from build123d import *

# Parameters (mm, degrees)
F0_W     = 457.2
F0_H     = 304.8
F0_R     = 1.8288
F0_R_2   = 41.34485
F1_DEPTH = 12.7
F2_W     = 144.399
F2_H     = 82.042
F3_DEPTH = 3.175
F4_R     = 1.5875
F5_DEPTH = 3.175


with BuildPart() as f1:
    # F0 (on Top) → F1 (new body)
    with BuildSketch(Plane.XY):
        Rectangle(F0_W, F0_H)
        with Locations((-186.120166, -107.938549)):
            Circle(F0_R, mode=Mode.SUBTRACT)
        with Locations((-98.490166, -107.938549)):
            Circle(F0_R, mode=Mode.SUBTRACT)
        with Locations((-142.305166, -64.123549)):
            Circle(F0_R_2, mode=Mode.SUBTRACT)
        with Locations((-186.120166, -20.308549)):
            Circle(F0_R, mode=Mode.SUBTRACT)
        with Locations((-98.490166, -20.308549)):
            Circle(F0_R, mode=Mode.SUBTRACT)
        with Locations((98.490166, -107.938549)):
            Circle(F0_R, mode=Mode.SUBTRACT)
        with Locations((186.120166, -107.938549)):
            Circle(F0_R, mode=Mode.SUBTRACT)
        with Locations((98.490166, -20.308549)):
            Circle(F0_R, mode=Mode.SUBTRACT)
        with Locations((142.305166, -64.123549)):
            Circle(F0_R_2, mode=Mode.SUBTRACT)
        with Locations((186.120166, -20.308549)):
            Circle(F0_R, mode=Mode.SUBTRACT)
        with Locations((-186.120166, 20.308549)):
            Circle(F0_R, mode=Mode.SUBTRACT)
        with Locations((-142.305166, 64.123549)):
            Circle(F0_R_2, mode=Mode.SUBTRACT)
        with Locations((-98.490166, 20.308549)):
            Circle(F0_R, mode=Mode.SUBTRACT)
        with Locations((-186.120166, 107.938549)):
            Circle(F0_R, mode=Mode.SUBTRACT)
        with Locations((-98.490166, 107.938549)):
            Circle(F0_R, mode=Mode.SUBTRACT)
        with Locations((98.490166, 20.308549)):
            Circle(F0_R, mode=Mode.SUBTRACT)
        with Locations((186.120166, 20.308549)):
            Circle(F0_R, mode=Mode.SUBTRACT)
        with Locations((142.305166, 64.123549)):
            Circle(F0_R_2, mode=Mode.SUBTRACT)
        with Locations((98.490166, 107.938549)):
            Circle(F0_R, mode=Mode.SUBTRACT)
        with Locations((186.120166, 107.938549)):
            Circle(F0_R, mode=Mode.SUBTRACT)
    extrude(amount=F1_DEPTH)

    # F2 (on face) → F3 (cut)
    with BuildSketch(Plane.XY.offset(12.7)):
        Rectangle(F2_W, F2_H)
    extrude(amount=-F3_DEPTH, mode=Mode.SUBTRACT)

    # F4 (on face) → F5 (cut, through all)
    with BuildSketch(Plane.XY.offset(12.7)):
        with Locations((-72.1995, 41.021)):
            Circle(F4_R)
        with Locations((72.1995, 41.021)):
            Circle(F4_R)
        with Locations((72.1995, -41.021)):
            Circle(F4_R)
        with Locations((-72.1995, -41.021)):
            Circle(F4_R)
    extrude(amount=-F5_DEPTH, mode=Mode.SUBTRACT)


solid = f1.part
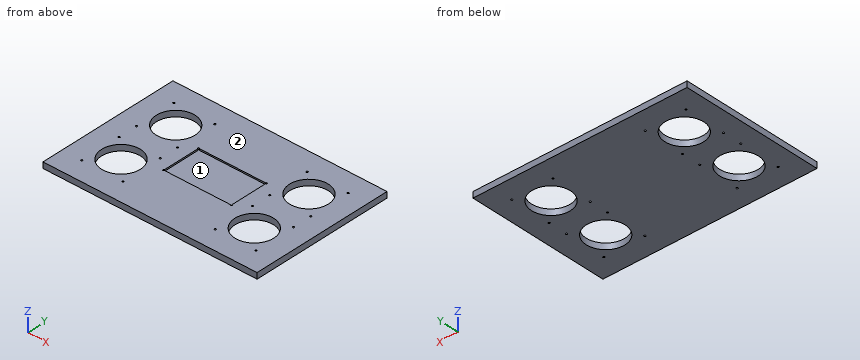
Work out the finished part from the listing and answer in its coordinate system (mm). Face numbers are marked on the shaded views. Give positions to 0.01 mm unless a question says otherwise; leave off trailing zeros. Write each loop counter-clockwise with the first axis right and the second up, starting at its lowest first coordinate (ties: lowest second). Pieces come first, ordered by that corner, then holes. Notation, with made-up numbers: (-33.75, 44.5) - (-23.75, 44.5) arc R28 cw to (-23.75, 78.5) - close; hole circle Ø10 at (55.5, 1). An arc over 180 degrees is marked (long way). One line per item, written item: value. Start each with the question number.
1. Find section D-D (z = 3.75). State how many separate pieces and enclosed holes the cut face has, then the cut area to 3 significant figures.
2. Find section C-C (y = 7). Write down the section's boundary in (x, z) (1 decimal).
3. Find section B-B (x = -23). Write down the section's boundary in (y, z) (3 decimals).
4. Consider probe 1 along Y at (x, z) = (99, 1.75); probe 2 along X at (y, z) = (62, 11.75); probe 3 along X at (y, z) = (-52, 6.5). Determine where each line is inside the solid, lowest interval first.
5. For a pull along X with two mould halves and no side action, classify the marked faces 1 and 2 as +X half, -X half, draft (parallel to the pull), parting line (faces both ways), or undercut.
6. Find section A-A (y = -75.5). Write down the section's boundary in (x, z), then the cut area to 3 significant figures.
Geometry results:
1. separate pieces: 1
1. enclosed holes: 20
1. area: 118,000 mm2
2. outline: (-228.6, 0) - (228.6, 0) - (228.6, 12.7) - (72.2, 12.7) - (72.2, 9.5) - (-72.2, 9.5) - (-72.2, 12.7) - (-228.6, 12.7) - close
3. outline: (-152.4, 0) - (152.4, 0) - (152.4, 12.7) - (41.021, 12.7) - (41.021, 9.525) - (-41.021, 9.525) - (-41.021, 12.7) - (-152.4, 12.7) - close
4. probe 1: -152.4 to -109.69, -106.18 to -22.06, -18.55 to 18.55, 22.06 to 106.18, 109.69 to 152.4
4. probe 2: -228.6 to -183.6, -101.01 to 101.01, 183.6 to 228.6
4. probe 3: -228.6 to -181.83, -102.78 to 102.78, 181.83 to 228.6
5. face 1: undercut
5. face 2: draft
6. outline: (-228.6, 0) - (-182.05, 0) - (-182.05, 12.7) - (-228.6, 12.7) - close; (-102.56, 0) - (102.56, 0) - (102.56, 12.7) - (-102.56, 12.7) - close; (182.05, 0) - (228.6, 0) - (228.6, 12.7) - (182.05, 12.7) - close
6. area: 3,790 mm2
